Check sheet for the modelled part. Datum: model origin and axes. Units: mm. Give positions to 0.01 mm unless a question says otherwise; leave off trailing zeros. Order: outer loops, then holes, each group sorted by start corner. A loop starts at its lowest first (then second) coordinate and runs counter-clockwise, first axis right, second up. Notation, with made-up numbers: M 81.25,68 L 138.25,68 A8 ccw 138.25,81 Z; hole C -0.5,83.25 d7. An arc over 180 degrees is marked long. One line per question, with ' | ' between items. Start each with the question number.
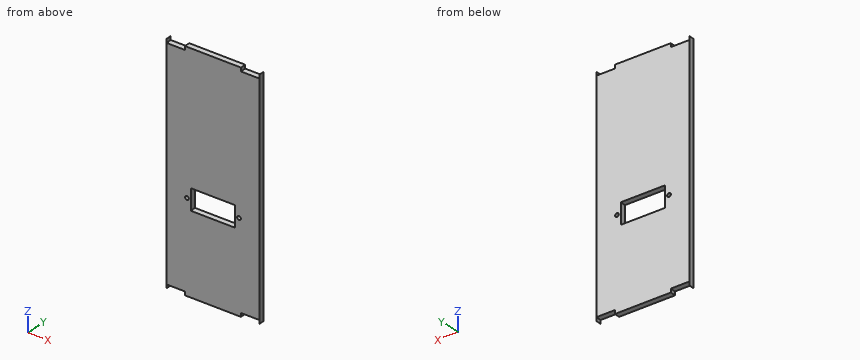
```python
from build123d import *

# Parameters (mm, degrees)
EXTRUDE_1_DEPTH     = 127
SKETCH_3_W          = 9.917998233
SKETCH_3_H          = 2
CUT_EXTRUDE_1_DEPTH = 890.48684692
SKETCH_4_R          = 1
SKETCH_4_W          = 23.8
SKETCH_4_H          = 11.5
CUT_EXTRUDE_2_DEPTH = 890.48684692


with BuildPart() as part:
    # 草图2 → 凸台-拉伸1 (new body)
    with BuildSketch(Plane(origin=(0, 0, 762.01), x_dir=(-1, 0, 0), z_dir=(0, 0, -1))):
        Polygon((-21.370258024, -5.639890041), (28.594871448, -7.506929626), (28.475974915, -10.504572636), (-21.489154557, -8.637533051), align=None)
    extrude(amount=-EXTRUDE_1_DEPTH)

    # 草图3 → 切除-拉伸1 (cut, through all)
    with BuildSketch(Plane(origin=(0.240248379, -6.429451979, 0), x_dir=(0.9993025894470269, 0.03734079169577059, 0), z_dir=(-0.03734079169577059, 0.9993025894470269, 0))):
        with Locations((-23.814242896, -763.01)):
            Rectangle(SKETCH_3_W, SKETCH_3_H)
        with Locations((16.185757105, -763.01)):
            Rectangle(SKETCH_3_W, SKETCH_3_H)
        with Locations((-23.814242896, -888.01)):
            Rectangle(SKETCH_3_W, SKETCH_3_H)
        with Locations((16.185757105, -888.01)):
            Rectangle(SKETCH_3_W, SKETCH_3_H)
    extrude(amount=-CUT_EXTRUDE_1_DEPTH, mode=Mode.SUBTRACT)

    # 草图4 → 切除-拉伸2 (cut, through all)
    with BuildSketch(Plane(origin=(0.240248379, -6.429451979, 0), x_dir=(0.9993025894470269, 0.03734079169577059, 0), z_dir=(-0.03734079169577059, 0.9993025894470269, 0))):
        with Locations(Location((10.144756221, -812.01, 0), (0, 0, 180))):
            Circle(SKETCH_4_R)
        with Locations((-17.855243779, -812.01)):
            Circle(SKETCH_4_R)
        with Locations((-3.855243779, -812.01)):
            Rectangle(SKETCH_4_W, SKETCH_4_H)
    extrude(amount=-CUT_EXTRUDE_2_DEPTH, mode=Mode.SUBTRACT)


solid = part.part
```
Item 1: Section check A-A, the plane x = -13. Record the cut outline in (y, z), then the cut area to 3 significant figures.
Item 2: Go/stop test with flat-tipped pins: P1, Ø5, axis at x = 3, z = 786, coming from the +Y side; P2, Ø1, axis at y = -7, z = 871.5, coming from the +X side; P3, Ø2.5, axis at x = -25.5, y = -8, coming from the -Z side. Record where each tip stops, or that it passes through.
Item 3: Section check B-B, the plane z = 790.5. Record the cut outline in (x, y).
Item 4: Scan lines: probe 1 along Z at (x, y) = (4, -8.05); probe 2 along Z at (x, y) = (-21.5, -9.95); probe 3 along Z at (x, y) = (-18, -8.2). Record each from-to range of solid material in increasing order. Write a range as [from, to].
Item 5: Section check C-C, the plane x = -24. Record the cut outline in (y, z), then the cut area to 3 significant figures.
Reported:
1) outline: M -9.93,762.01 L -6.92,762.01 L -6.92,806.26 L -9.93,806.26 Z; M -9.93,817.76 L -6.92,817.76 L -6.92,889.01 L -9.93,889.01 Z | area: 347 mm^2
2) P1: stops at y = -6.23 | P2: stops at x = 21.44 | P3: stops at z = 764.01
3) outline: M -28.59,-7.51 L -28.48,-10.5 L 21.49,-8.64 L 21.37,-5.64 Z
4) probe 1: z = [762.01, 806.26], [817.76, 889.01] | probe 2: z = [764.01, 887.01] | probe 3: z = [762.01, 811.11], [812.91, 889.01]
5) outline: M -10.34,764.01 L -7.34,764.01 L -7.34,887.01 L -10.34,887.01 Z | area: 369 mm^2
